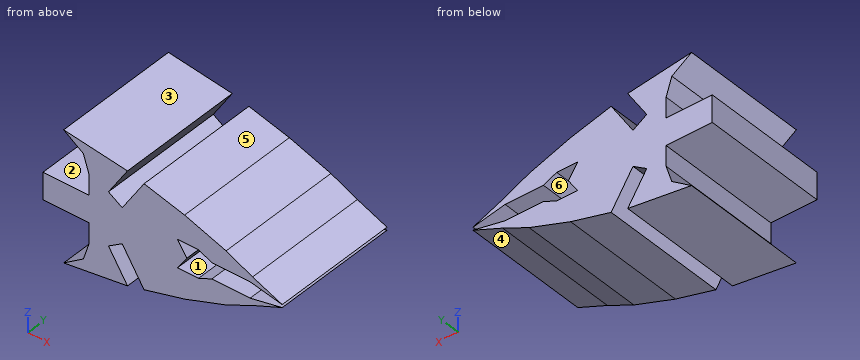
Autodesk Inventor part; units mm, degrees
ref_plane "YZ Plane" through (0, 0, 0) normal (1, 0, 0) x (0, 1, 0)
ref_plane "XZ Plane" through (0, 0, 0) normal (0, 1, 0) x (-1, 0, 0)
ref_plane "XY Plane" through (0, 0, 0) normal (0, 0, 1) x (1, 0, 0)
sketch "Sketch1" plane through (0, 0, 0) normal (0, 1, 0) x (-1, 0, 0)
  line L0 (-17.4285, 2.7736) -> (-12.1383, 5.2631)
  line L1 (-12.1383, 5.2631) -> (-3.84, 8.1675)
  line L2 (-3.84, 8.1675) -> (4.2592, 10.3027)
  line L3 (7.5702, 11.1757) -> (20.3289, 12.9391)
  line L4 (20.3289, 12.9391) -> (16.3872, 10.2421)
  line L5 (16.3872, 10.2421) -> (15.2462, 6.7153)
  line L6 (15.2462, 6.7153) -> (15.2462, 2.676)
  line L7 (15.2462, 2.676) -> (24.4575, 2.676)
  line L8 (24.4575, 2.676) -> (24.4575, 0)
  line L9 (-17.4285, 2.7736) -> (-23.3511, 0.2916)
  line L10 (24.4575, 0) -> (-4.2928, 0)
  line L11 (-17.4285, -2.7736) -> (-12.1383, -5.2631)
  line L12 (-12.1383, -5.2631) -> (-3.84, -8.1675)
  line L13 (-3.84, -8.1675) -> (4.2592, -10.3027)
  line L14 (7.5702, -11.1757) -> (20.3289, -12.9391)
  line L15 (20.3289, -12.9391) -> (16.3872, -10.2421)
  line L16 (16.3872, -10.2421) -> (15.2462, -6.7153)
  line L17 (15.2462, -6.7153) -> (15.2462, -2.676)
  line L18 (15.2462, -2.676) -> (24.4575, -2.676)
  line L19 (24.4575, -2.676) -> (24.4575, 0)
  line L20 (-17.4285, -2.7736) -> (-23.3511, -0.2916)
  line L21 (15.2462, -2.676) -> (15.2462, 2.676)
  line L22 (7.5702, 11.1757) -> (11.3708, 5.2631)
  line L23 (11.3708, 5.2631) -> (8.6308, 3.5018)
  line L24 (8.6308, 3.5018) -> (4.2592, 10.3027)
  line L25 (7.5702, -11.1757) -> (11.3708, -5.2631)
  line L26 (8.6308, -3.5018) -> (4.2592, -10.3027)
  line L27 (11.3708, -5.2631) -> (8.6308, -3.5018)
  line L28 (-9.2958, -1.5896) -> (-6.6168, -2.7736)
  line L29 (-6.6168, -2.7736) -> (-2.4179, -2.7736)
  line L30 (-2.4179, -2.7736) -> (-4.2928, 0)
  line L31 (-9.2958, 1.5896) -> (-6.6168, 2.7736)
  line L32 (-6.6168, 2.7736) -> (-2.4179, 2.7736)
  line L33 (-2.4179, 2.7736) -> (-4.2928, 0)
  line L34 (-9.2958, 1.5896) -> (-16.9323, 1.5896)
  line L35 (-23.3511, 0.2916) -> (-16.9323, 1.5896)
  line L36 (-9.2958, -1.5896) -> (-16.9323, -1.5896)
  line L37 (-23.3511, -0.2916) -> (-16.9323, -1.5896)
  point P0 (0, 0)
  point P1 (0, 0)
extrude "Extrusion1" add sketch "Sketch1" along normal blind 25.4
CAD build for the part. Positions are in the model's coordinates, mm. Face numbers are marked on the shaded views. A direction names the side the tool comes from. Round coordinates to 2 decimals unless told otherwise and drop trailing zeros. Loops run counter-clockwise (first coordinate to the right, second up) from the corner with the lowest first, then second, coordinate; pieces in that order, holes last.
(1) Cut at A-A (z = -9.5). Give the cut face in (x, y), plus the area to 3 significant figures.
(2) Wall check: line 1 along Z through (x, y) = (6, 4); line 2 along Z through (x, y) = (6.5, 13.5); line 3 along X through (y, z) = (6, -2). Give the ranges that are in metal, low to high.
(3) Drop flat-ended pins along their axis: pin 1 (1 mm diameter, centred on x = -1, z = 0, fed in from -Y); pin 2 (4.5 mm diameter, centred on x = 4, y = 18.5, fed in from -Z); pin 3 (10 mm diameter, centred on x = -7.5, y = 20.5, fed in from -Z); pin 4 (4 mm diameter, centred on x = 15, y = 7, fed in from +Z). Give the stop position or say it passes through.
(4) Cut at B-B (x = -10). Give the cut face in (y, z).
(5) Which spindle directions (+Z, -Z, +X, -X, +Y, -Y) get a long thin tool onto all of the face, cutting with end or side? Do the marked faces 1, 2 and 3. Say none if no direction does.
(6) Two-plate mould, pull along Z, no slides. Class the marked faces 4, 5 and 6: +Z half, -Z half, draft (parallel to the pull), parting line (faces both ways), or undercut.
(7) Cut at C-C (x = -1). Give the cut face in (y, z), plus the area to 3 significant figures.
Findings below:
1. outline: (-16.15, 0) - (-8.65, 0) - (-8.65, 25.4) - (-16.15, 25.4) - close; (-4.78, 0) - (-1.21, 0) - (-1.21, 25.4) - (-4.78, 25.4) - close
1. area: 281 mm2
2. line 1: z = -7.41 to -2.77, 2.77 to 7.41
2. line 2: z = -7.24 to -2.77, 2.77 to 7.24
2. line 3: x = -24.46 to 2.94, 8.37 to 19.27
3. pin 1: stops at y = 0
3. pin 2: stops at z = -8.72
3. pin 3: stops at z = -11.86
3. pin 4: stops at z = 4.86
4. outline: (0, -11.51) - (25.4, -11.51) - (25.4, -7.4) - (0, -7.4) - close; (0, -4.38) - (25.4, -4.38) - (25.4, 4.38) - (0, 4.38) - close; (0, 7.4) - (25.4, 7.4) - (25.4, 11.51) - (0, 11.51) - close
5. face 1: +Y, -Y
5. face 2: -X, +Y, -Y
5. face 3: +Z, +X, +Y, -Y
6. face 4: -Z half
6. face 5: +Z half
6. face 6: undercut
7. outline: (0, -9.44) - (25.4, -9.44) - (25.4, 9.44) - (0, 9.44) - close
7. area: 480 mm2
